from build123d import *

# Parameters (mm, degrees)
BOSS_EXTRUDE1_DEPTH = 8
SKETCH1_3_R         = 1.5
BOSS_EXTRUDE2_DEPTH = 3
BOSS_EXTRUDE5_START = -8
BOSS_EXTRUDE5_DEPTH = 8


with BuildPart() as part:
    # Sketch1 → Boss-Extrude1 (new body)
    with BuildSketch(Plane(origin=(0, 0, 0), x_dir=(0, 0, -1), z_dir=(1, 0, 0))):
        with BuildLine():
            ThreePointArc((-4.119669775, -1.65532903), (0.037822774, 4.439635423), (4.090869231, -1.725277422))
            Line((4.090869231, -1.725277422), (1.82908276, -24.946763134))
            Line((1.82908276, -24.946763134), (-2.312399702, -24.946763134))
            Line((-2.312399702, -24.946763134), (-4.119669775, -1.65532903))
        make_face()
        with BuildLine():
            Line((-3.575175872, -1.65532903), (-1.968294835, -22.364222709))
            Line((-1.968294835, -22.364222709), (1.531705165, -22.364222709))
            Line((1.531705165, -22.364222709), (3.541950668, -1.725277422))
            ThreePointArc((3.541950668, -1.725277422), (0.038719155, 3.939606268), (-3.575175872, -1.65532903))
        make_face(mode=Mode.SUBTRACT)
    extrude(amount=BOSS_EXTRUDE1_DEPTH)

    # Sketch1<3> → Boss-Extrude2 (add)
    with BuildSketch(Plane(origin=(0, 0, 0), x_dir=(0, 0, -1), z_dir=(1, 0, 0))):
        with BuildLine():
            ThreePointArc((-3.575175872, -1.65532903), (0.038719155, 3.939606268), (3.541950668, -1.725277422))
            Line((3.541950668, -1.725277422), (1.531705165, -22.364222709))
            Line((1.531705165, -22.364222709), (-1.968294835, -22.364222709))
            Line((-1.968294835, -22.364222709), (-3.575175872, -1.65532903))
        make_face()
        Circle(SKETCH1_3_R, mode=Mode.SUBTRACT)
    extrude(amount=BOSS_EXTRUDE2_DEPTH)

    # Sketch4 → Boss-Extrude5 (add)
    with BuildSketch(Plane(origin=(8, 0, 0), x_dir=(0, 0, -1), z_dir=(1, 0, 0)).offset(BOSS_EXTRUDE5_START)):
        with BuildLine():
            Line((4.439796532, 5.000361233), (-4.439796532, 5.000361233))
            Line((-4.439796532, 5.000361233), (-4.439796532, -2e-08))
            ThreePointArc((-4.439796532, -2e-08), (1e-08, 4.439796532), (4.439796532, -4e-08))
            Line((4.439796532, -4e-08), (4.439796532, 5.000361233))
        make_face()
        with BuildLine():
            ThreePointArc((-4.119669775, -1.65532903), (-4.359030213, -0.842999912), (-4.439796532, -2e-08))
            Line((-4.439796532, -2e-08), (-4.439796532, -42.946763134))
            Line((-4.439796532, -42.946763134), (4.439796532, -42.946763134))
            Line((4.439796532, -42.946763134), (4.439796532, -4e-08))
            ThreePointArc((4.439796532, -4e-08), (4.351690488, -0.880104054), (4.090869231, -1.725277422))
            Line((4.090869231, -1.725277422), (1.82908276, -24.946763134))
            Line((1.82908276, -24.946763134), (-2.312399702, -24.946763134))
            Line((-2.312399702, -24.946763134), (-4.119669775, -1.65532903))
        make_face()
    extrude(amount=BOSS_EXTRUDE5_DEPTH)


solid = part.part
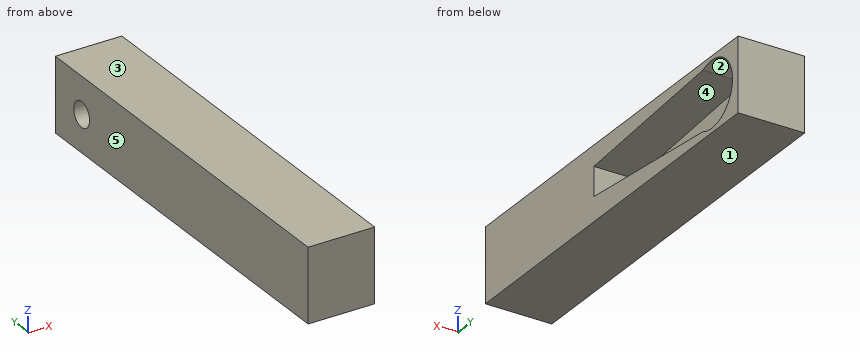
The listing builds one solid part. Answer for the finished solid, in the listing's coordinates (mm). Face numbers are marked on the shaded views. A direction names the side the tool comes from. Round coordinates to 2 decimals unless told otherwise and drop trailing zeros. Loops run counter-clockwise (first coordinate to the right, second up) from the corner with the lowest first, then second, coordinate; pieces in that order, holes last. Notation, with made-up numbers: M 42.5,75 L 94.5,75 A29 ccw 94.5,111 Z; hole C 5.5,62.25 d11. An arc over 180 degrees is marked long. Write each question's results on one line, items separated by ' | '. Start each with the question number.
1) Find section D-D on y = -16. Write down the section's boundary in (x, z), plus the area to 3 significant figures.
2) Straight lines are drawn through the part: probe 1 along Y at (x, z) = (1.9, 0); probe 2 along Y at (x, z) = (4.65, 0); probe 3 along Z at (x, y) = (5.15, 0). For each, find the intervals that lie inside material, in ascending order.
3) Determine the mould class of the marked faces 1, 2 and 3 for opening direction Z: pulls with the +Z half, pulls with the -Z half, needs draft (parallel to the pull), parting line crosses it, or undercut.
4) Find section B-B on z = 0. Write down the section's boundary in (x, y).
5) Find section C-C on x = 6.75. Write down the section's boundary in (y, z).
6) Find section A-A on y = 0. Write down the section's boundary in (x, z), plus the area to 3 significant figures.
7) Which of the six approach directions +Z, -Z, +X, -X, +Y, -Y give full straight-line access (tool end or side, diameter ignored) to the marked faces 4 and 5?
Final values:
1) outline: M 0,-4.44 L 8,-4.44 L 8,-2.15 L 3,-2.15 L 3,2.46 L 8,2.46 L 8,4.44 L 0,4.44 Z | area: 48.0 mm²
2) probe 1: -42.95 to -1.5, 1.5 to 5 | probe 2: -42.95 to -22.36, 3.94 to 5 | probe 3: -4.44 to -3.94, 3.94 to 4.44
3) face 1: pulls with the -Z half | face 2: undercut | face 3: pulls with the +Z half
4) outline: M 0,-42.95 L 8,-42.95 L 8,-22.36 L 3,-22.36 L 3,-1.5 L 0,-1.5 Z; M 0,1.5 L 3,1.5 L 3,3.94 L 8,3.94 L 8,5 L 0,5 Z
5) outline: M -42.95,-4.44 L 5,-4.44 L 5,4.44 L -42.95,4.44 Z; hole M -22.36,-1.53 L -1.73,-3.54 A3.94 ccw long -1.66,3.58 L -22.36,1.97 Z
6) outline: M 0,-4.44 L 8,-4.44 L 8,-3.94 L 3,-3.94 L 3,-1.5 L 0,-1.5 Z; M 0,1.5 L 3,1.5 L 3,3.94 L 8,3.94 L 8,4.44 L 0,4.44 Z | area: 22.6 mm²
7) face 4: +X | face 5: +Z, -Z, -X, +Y, -Y
